The figure shows three views and two pictorial views of one solid part (mm, origin at its lowest corner). Answer the questions. A direction names the side the tool comes from. Round coordinates to 2 decimals unless told otherwise and drop trailing zeros. Order: outer loops, then holes, each group sorted by start corner. A loop starts at its lowest first (then second) coordinate and runs counter-clockwise, first axis right, second up. Notation, with made-up numbers: (-40, 42) - (-14, 42) arc R28 cw to (-14, 64) - close; hole circle Ø8 at (67, 7). An arc over 180 degrees is marked (long way). Use CSV: the item, a comma, the result in double quotes.
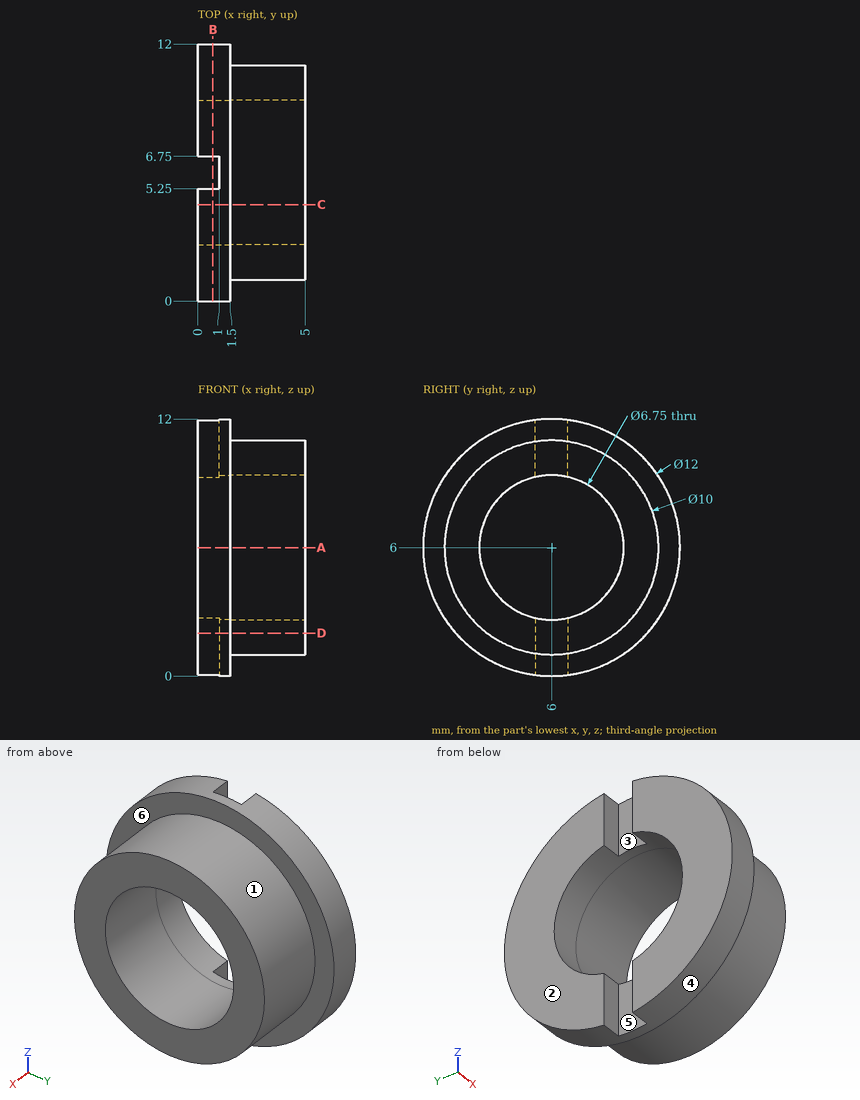
(1) Find section B-B (x = 0.7). Determine the outline of the cut face in (y, z) (3 decimals).
Findings below:
outline,"(5.25, 0.047) - (5.25, 2.709) arc R3.375 cw to (5.25, 9.291) - (5.25, 11.953) arc R6 ccw to start; (6.75, 0.047) arc R6 ccw to (6.75, 11.953) - (6.75, 9.291) arc R3.375 cw to (6.75, 2.709) - close"
(2) For the marked faces 1, 2 and 3, determine the directions among +Z, -Z, +X, -X, +Y, -Y from which every point of the face is accessible in a straight line to the end or side of a thin tool.
Findings below:
face 1,"+X"
face 2,"+Z, -Z, -X, +Y, -Y"
face 3,"+Z, -Z, -X"
(3) Find section A-A (z = 6). Determine the outline of the cut face in (x, y) (3 decimals).
Findings below:
outline,"(0, 0) - (1.5, 0) - (1.5, 1) - (5, 1) - (5, 2.625) - (0, 2.625) - close; (0, 9.375) - (5, 9.375) - (5, 11) - (1.5, 11) - (1.5, 12) - (0, 12) - close"
(4) Each of these flat-tipped pins is pushed along its axis until it touches: pin 1 (0.5 mm diameter, centred on x = 0.5, z = 11, fed in from -Y); pin 2 (0.8 mm diameter, centred on y = 6, z = 1.5, fed in from -X); pin 3 (1.1 mm diameter, centred on x = 0.5, z = 10, fed in from +Y); pin 4 (4 mm diameter, centred on y = 6, z = 6, fed in from -X). Where does it stop, or does it pass through?
Findings below:
pin 1,"stops at y = 2.33"
pin 2,"stops at x = 1"
pin 3,"stops at y = 10.91"
pin 4,"passes through"
(5) Find the intervals of material crossed by L1, parallel to Y at x = 1.1, z = 6 (3 decimals); L2, parallel to Y at x = 2.6, z = 6 (3 decimals); L3, parallel to X at y = 9.25, z = 10.5, in increasing order. Write a range as from..to.
Findings below:
L1,"y = 0..2.625, 9.375..12"
L2,"y = 1..2.625, 9.375..11"
L3,"x = 0..1.5"
(6) Find section C-C (y = 4.5). Determine the outline of the cut face in (x, z).
Findings below:
outline,"(0, 0.19) - (1.5, 0.19) - (1.5, 1.23) - (5, 1.23) - (5, 2.98) - (0, 2.98) - close; (0, 9.02) - (5, 9.02) - (5, 10.77) - (1.5, 10.77) - (1.5, 11.81) - (0, 11.81) - close"
(7) Find section D-D (z = 2). Determine the outline of the cut face in (x, y), and give its area (3 significant figures).
Findings below:
outline,"(0, 1.53) - (1.5, 1.53) - (1.5, 3) - (5, 3) - (5, 9) - (1.5, 9) - (1.5, 10.47) - (0, 10.47) - (0, 6.75) - (1, 6.75) - (1, 5.25) - (0, 5.25) - close"
area,"32.9 mm²"
(8) The mould has two halves that part along Y. Classify the marked faces 4, 5 and 6: released by +Y, released by -Y, zero draft, split by the parting line, or undercut.
Findings below:
face 4,"split by the parting line"
face 5,"undercut"
face 6,"zero draft"
